from build123d import *

# Parameters (mm, degrees)
SKETCH2_W           = 6.35
SKETCH2_H           = 17.145
BOSS_EXTRUDE1_DEPTH = 6.35
CUT_EXTRUDE1_DEPTH  = 135.924052271
FILLET1_R           = 2.54
FILLET2_R           = 1.27


with BuildPart() as part:
    # Sketch2 → Boss-Extrude1 (new body)
    with BuildSketch(Plane.XY):
        Polygon((98.425, 84.7725), (-98.425, 84.7725), (-98.425, 67.6275), (-98.425, 8.5725), (-98.425, -8.5725), (-98.425, -67.6275), (-98.425, -84.7725), (98.425, -84.7725), (98.425, -67.6275), (98.425, -8.5725), (98.425, 8.5725), (98.425, 67.6275), align=None)
        with Locations((-101.6, 76.2)):
            Rectangle(SKETCH2_W, SKETCH2_H)
        with Locations((-101.6, 0)):
            Rectangle(SKETCH2_W, SKETCH2_H)
        with Locations((101.6, 76.2)):
            Rectangle(SKETCH2_W, SKETCH2_H)
        with Locations((101.6, 0)):
            Rectangle(SKETCH2_W, SKETCH2_H)
        with Locations((101.6, -76.2)):
            Rectangle(SKETCH2_W, SKETCH2_H)
        with Locations((-101.6, -76.2)):
            Rectangle(SKETCH2_W, SKETCH2_H)
    extrude(amount=BOSS_EXTRUDE1_DEPTH)

    # Sketch3 → Cut-Extrude1 (cut, through all)
    with BuildSketch(Plane.XY.offset(6.35)):
        Polygon((-9.72090457, 0), (-85.725, 63.899739491), (-85.725, -63.899739491), align=None)
        Polygon((76.00409543, 72.0725), (-76.00409543, 72.0725), (0, 8.172760509), align=None)
        Polygon((85.725, -63.899739491), (85.725, 63.899739491), (9.72090457, 0), align=None)
        Polygon((0, -8.172760509), (-76.00409543, -72.0725), (76.00409543, -72.0725), align=None)
    extrude(amount=-CUT_EXTRUDE1_DEPTH, mode=Mode.SUBTRACT)

    # Fillet1
    fillet1_edges = [part.edges().sort_by_distance(p)[0] for p in [
        (85.725, 63.899739491, 3.175),
        (85.725, -63.899739491, 3.175),
        (9.72090457, 0, 3.175),
        (76.00409543, 72.0725, 3.175),
        (0, 8.172760509, 3.175),
        (-76.00409543, 72.0725, 3.175),
        (0, -8.172760509, 3.175),
        (76.00409543, -72.0725, 3.175),
        (-76.00409543, -72.0725, 3.175),
        (-9.72090457, 0, 3.175),
        (-85.725, -63.899739491, 3.175),
        (-85.725, 63.899739491, 3.175),
    ]]
    fillet(fillet1_edges, radius=FILLET1_R)

    # Fillet2
    fillet2_edges = [part.edges().sort_by_distance(p)[0] for p in [
        (104.775, 8.5725, 3.175),
        (104.775, -8.5725, 3.175),
        (104.775, -67.6275, 3.175),
        (104.775, -84.7725, 3.175),
        (-104.775, -8.5725, 3.175),
        (-104.775, 8.5725, 3.175),
        (-104.775, 67.6275, 3.175),
        (-104.775, 84.7725, 3.175),
        (104.775, 84.7725, 3.175),
        (104.775, 67.6275, 3.175),
        (-104.775, -67.6275, 3.175),
        (-104.775, -84.7725, 3.175),
    ]]
    fillet(fillet2_edges, radius=FILLET2_R)


solid = part.part
Read the model definition and answer for the solid it produces. Units are mm, in the model's axes. A direction names the side the tool comes from. Round coordinates to 2 decimals unless told otherwise and drop trailing zeros. Order: outer loops, then holes, each group sorted by start corner. A loop starts at its lowest first (then second) coordinate and runs counter-clockwise, first axis right, second up. Notation, with made-up numbers: (-36.5, 22.5) - (-22.5, 22.5) arc R28 ccw to (-22.5, 54.5) - close; hole circle Ø5 at (42, -10.75). An arc over 180 degrees is marked (long way). Use one line per item in the form item = value. Start each with the question number.
(1) The part is cut by section B-B (y = 13.5). Give the vertices of the cut face in (x, z) (3 decimals), then the cut area to 3 significant figures.
(2) A flat-ended cylindrical pin translates along its axis: pin 1 Ø3 at (y, z) = (37.5, 3.5) entering from -X (3 decimals). Find the tip coordinate at first contact, or state that the pin passes through.
(3) Determine the mould class of faces 1 (the face through (1, 84.773, 3)), 2 (the face through (-1, -84.773, 3)), 3 (the face through (98.425, -39, 3)) for opening direction Y: +Y half, -Y half, draft (parallel to the pull), parting line (faces both ways), or undercut.
(4) The part is cut by section C-C (z = 2). Count the separate pieces of the cut face and the enclosed holes in it, then the cut area to 3 significant figures.
(5) Find the intervals of material crossed by line 1 along X through (y, z) = (-59.5, 2.75) (3 decimals); line 2 along Y through (x, z) = (11, 3.5); line 3 along X through (y, z) = (69.5, 3) (3 decimals), in increasing order. Write a range as from..to.
(6) The part is cut by section A-A (x = 19.5). Give the vertices of the cut face in (y, z), then the cut area to 3 significant figures.
(7) For faces 4 (the face through (-101, -67.628, 3)), 5 (the face through (1, 72.072, 3)), 6 (the face through (98.425, 38, 3)), determine the directions among +Z, -Z, +X, -X, +Y, -Y from which every point of the face is accessible in a straight line to the end or side of a thin tool.
Checked values:
q1.outline = (-98.425, 0) - (-85.725, 0) - (-85.725, 6.35) - (-98.425, 6.35) - close; (-25.778, 0) - (-6.336, 0) - (-6.336, 6.35) - (-25.778, 6.35) - close; (6.336, 0) - (25.778, 0) - (25.778, 6.35) - (6.336, 6.35) - close; (85.725, 0) - (98.425, 0) - (98.425, 6.35) - (85.725, 6.35) - close
q1.area = 408 mm^2
q2.pin_1 = -98.425
q3.face_1 = +Y half
q3.face_2 = -Y half
q3.face_3 = undercut
q4.separate_pieces = 1
q4.enclosed_holes = 4
q4.area = 14,700 mm^2
q5.line_1 = -98.425..-85.496, -80.492..-61.05, 61.05..80.492, 85.496..98.425
q5.line_2 = -84.77..-72.07, -17.42..17.42, 72.07..84.77
q5.line_3 = -104.775..-71.576, 71.576..104.775
q6.outline = (-84.77, 0) - (-72.07, 0) - (-72.07, 6.35) - (-84.77, 6.35) - close; (-24.57, 0) - (-8.22, 0) - (-8.22, 6.35) - (-24.57, 6.35) - close; (8.22, 0) - (24.57, 0) - (24.57, 6.35) - (8.22, 6.35) - close; (72.07, 0) - (84.77, 0) - (84.77, 6.35) - (72.07, 6.35) - close
q6.area = 369 mm^2
q7.face_4 = +Z, -Z, -X
q7.face_5 = +Z, -Z
q7.face_6 = +Z, -Z, +X
